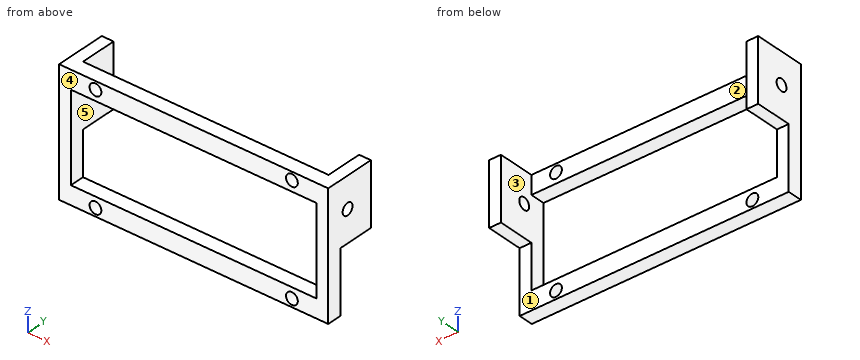
from build123d import *

# Parameters (mm, degrees)
SKETCH_1_W          = 62.5
SKETCH_1_H          = 4.7
SKETCH_1_R          = 1.5
EXTRUDE_1_DEPTH     = 3.7
SKETCH_2_W          = 31.8
SKETCH_2_H          = 3.7
EXTRUDE_2_DEPTH     = 3
SKETCH_3_W          = 3
SKETCH_3_H          = 15.9
EXTRUDE_3_DEPTH     = 13
SKETCH_4_R          = 1.5
CUT_EXTRUDE_1_DEPTH = 13


with BuildPart() as part:
    # 草图1 → 凸台-拉伸1 (new body)
    with BuildSketch(Plane(origin=(0, 0, 0), x_dir=(1, 0, 0), z_dir=(0, 1, 0))):
        Rectangle(SKETCH_1_W, SKETCH_1_H)
        with Locations((25, 0.3)):
            Circle(SKETCH_1_R, mode=Mode.SUBTRACT)
        with Locations((-25, 0.3)):
            Circle(SKETCH_1_R, mode=Mode.SUBTRACT)
    extrude_1 = extrude(amount=EXTRUDE_1_DEPTH)

    # 草图2 → 凸台-拉伸2 (add)
    with BuildSketch(Plane.ZY.offset(31.25)):
        with Locations((13.55, 1.85)):
            Rectangle(SKETCH_2_W, SKETCH_2_H)
    extrude_2 = extrude(amount=EXTRUDE_2_DEPTH)

    # 镜向1: 凸台-拉伸2 across plane
    add(extrude_2.mirror(Plane(origin=(0, 0, 0), x_dir=(0, 0, 1), z_dir=(1, 0, 0))))

    # 镜向2: 凸台-拉伸1 across plane
    add(extrude_1.mirror(Plane.XY.offset(13.55)))

    # 草图3 → 凸台-拉伸3 (add)
    with BuildSketch(Plane.XZ):
        with Locations((-32.75, 21.5)):
            Rectangle(SKETCH_3_W, SKETCH_3_H)
    extrude_3 = extrude(amount=-EXTRUDE_3_DEPTH)

    # 草图4 → 切除-拉伸1 (cut)
    with BuildSketch(Plane.ZY.offset(34.25)):
        with Locations((21.592743177, 5.9)):
            Circle(SKETCH_4_R)
    cut_extrude_1 = extrude(amount=-CUT_EXTRUDE_1_DEPTH, mode=Mode.SUBTRACT)

    # 镜向3: 凸台-拉伸3, 切除-拉伸1 across plane
    add(extrude_3.mirror(Plane(origin=(0, 0, 0), x_dir=(0, 0, 1), z_dir=(1, 0, 0))))
    add(cut_extrude_1.mirror(Plane(origin=(0, 0, 0), x_dir=(0, 0, 1), z_dir=(1, 0, 0))), mode=Mode.SUBTRACT)


solid = part.part
Geometry check sheet. Reference: the model listing, model coordinates, mm. Face numbers are marked on the shaded views. A direction names the side the tool comes from. Round coordinates to 2 decimals unless told otherwise and drop trailing zeros. Loops run counter-clockwise (first coordinate to the right, second up) from the corner with the lowest first, then second, coordinate; pieces in that order, holes last. Notation, with made-up numbers: (66.5, -8) -> (76.5, -8) arc R27 ccw to (76.5, 24) -> close; hole circle Ø4 at (88, 21.25). An arc over 180 degrees is marked (long way). Answer as a JSON object with one key per item and string values. Group by question number.
Item 1: Cross-section at C-C, the plane z = 10. Record the cut outline in (x, y), plus the area to 3 significant figures.
Item 2: Thickness scan on line 1 along Z through (x, y) = (-25, 2.6); line 2 along X through (y, z) = (1.4, -0.3); line 3 along X through (y, z) = (6, 28). Record the ranges inside material, lowest first.
Item 3: Set-up check for the marked faces 1, 2 and 3: record each of +Z, -Z, +X, -X, +Y, -Y from which the full face is reachable in a straight line by a thin tool's end or side.
Item 4: Cross-section at D-D, the plane x = -5. Record the cut outline in (y, z), plus the area to 3 significant figures.
Item 5: Cross-section at A-A, the plane x = -25. Record the cut outline in (y, z), plus the area to 3 significant figures.
Item 6: Depth check by flat-ended pin: pin 1 Ø4 at (x, z) = (-0.5, 26) entering from +Y; pin 2 Ø1.5 at (x, y) = (-33, 9.5) entering from -Z. Enter the tip coordinate at first touch or a pass-through.
Item 7: Release check for a two-part mould opening along Z. For the marked faces 4 and 5 record: pulls with the +Z half, pulls with the -Z half, needs draft (parallel to the pull), parting line crosses it, or undercut.
Item 8: Cross-section at B-B, the plane z = 27.4. Record the cut outline in (x, y), plus the area to 3 significant figures.
Determined:
{
 "1": {"outline": "(-34.25, 0) -> (-31.25, 0) -> (-31.25, 3.7) -> (-34.25, 3.7) -> close; (31.25, 0) -> (34.25, 0) -> (34.25, 3.7) -> (31.25, 3.7) -> close", "area": "22.2 mm²"},
 "2": {"line 1": "z = -2.35 to -1.8, 1.2 to 2.35, 24.75 to 25.9, 28.9 to 29.45", "line 2": "x = -34.25 to -26.5, -23.5 to 23.5, 26.5 to 34.25", "line 3": "x = -34.25 to -31.25, 31.25 to 34.25"},
 "3": {"face 1": "-Z, +X, -X, +Y", "face 2": "+Z, -Z, +Y", "face 3": "+Y"},
 "4": {"outline": "(0, -2.35) -> (3.7, -2.35) -> (3.7, 2.35) -> (0, 2.35) -> close; (0, 24.75) -> (3.7, 24.75) -> (3.7, 29.45) -> (0, 29.45) -> close", "area": "34.8 mm²"},
 "5": {"outline": "(0, -2.35) -> (3.7, -2.35) -> (3.7, -1.8) -> (0, -1.8) -> close; (0, 1.2) -> (3.7, 1.2) -> (3.7, 2.35) -> (0, 2.35) -> close; (0, 24.75) -> (3.7, 24.75) -> (3.7, 25.9) -> (0, 25.9) -> close; (0, 28.9) -> (3.7, 28.9) -> (3.7, 29.45) -> (0, 29.45) -> close", "area": "12.6 mm²"},
 "6": {"pin 1": "stops at y = 3.7", "pin 2": "stops at z = 13.55"},
 "7": {"face 4": "needs draft", "face 5": "undercut"},
 "8": {"outline": "(-34.25, 0) -> (-26.5, 0) -> (-26.5, 3.7) -> (-31.25, 3.7) -> (-31.25, 13) -> (-34.25, 13) -> close; (-23.5, 0) -> (23.5, 0) -> (23.5, 3.7) -> (-23.5, 3.7) -> close; (26.5, 0) -> (34.25, 0) -> (34.25, 13) -> (31.25, 13) -> (31.25, 3.7) -> (26.5, 3.7) -> close", "area": "287 mm²"}
}
